from build123d import *

# Parameters (mm, degrees)
F0_W     = 254
F0_H     = 254
F1_DEPTH = 82.87358
F4_R     = 13.060022
F5_DEPTH = 44.433


with BuildPart() as f1:
    # F0 (on Top) → F1 (new body)
    with BuildSketch(Plane.XY):
        Rectangle(F0_W, F0_H)
    extrude(amount=F1_DEPTH)


with BuildPart() as f3:
    # F2 (on Right) → F3 (revolve)
    with BuildSketch(Plane.YZ):
        Polygon((-27.195146, 7.24093), (-35.484381, 0), (42.802874, 0), (42.802874, 21.363337), (-8.774616, 21.363337), (-14.914793, 7.24093), align=None)
    revolve(axis=Axis((0, 3.659246, 0), (0, -1, 0)))


with BuildPart() as f5_tool:
    # F4 (on face) → F5 (new body)
    with BuildSketch(Plane(origin=(0, 42.802874, 0), x_dir=(-1, 0, 0), z_dir=(0, 1, 0))):
        Circle(F4_R)
    extrude(amount=-F5_DEPTH)


with BuildPart() as f1_1:
    add(f1.part)

    # F5: cut by f5_tool
    add(f5_tool.part, mode=Mode.SUBTRACT)


with BuildPart() as f3_1:
    add(f3.part)

    # F5: cut by f5_tool
    add(f5_tool.part, mode=Mode.SUBTRACT)


with BuildPart() as f1_2:
    add(f1_1.part)

    # F6: intersect F3
    add(f3_1.part, mode=Mode.INTERSECT)


solid = f1_2.part
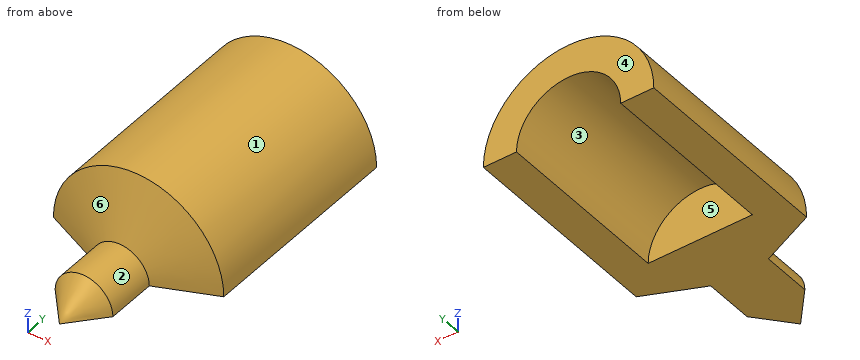
Verification items for the finished model (mm, model axes). Face numbers are marked on the shaded views. A direction names the side the tool comes from. Give positions to 0.01 mm unless a question says otherwise; leave off trailing zeros. Write each loop counter-clockwise with the first axis right and the second up, starting at its lowest first coordinate (ties: lowest second). Pieces come first, ordered by that corner, then holes.
(1) Cross-section at A-A (x = 0). Enter the section's corners in (y, z).
(2) Access from +Z, -Z, +X, -X, +Y, -Y to the whole of each face (thin tool, end or side, straight path). Record for the marked faces 1, 2 and 3.
(3) Gauge pin test, flat ends, axial feed: pin 1 (12 mm diameter, centred on x = 10, y = 2, fed in from +Z); pin 2 (2 mm diameter, centred on y = -12, z = 4, fed in from +X); pin 3 (6 mm diameter, centred on x = 0, z = 14.5, fed in from -Y). Record the tip position at first contact, or that the pin passes through.
(4) Material ranges on line 1 (X direction, y = 27.5, z = 11.5); line 2 (X direction, y = 34, z = 7.5); line 3 (X direction, y = -28.5, z = 5), recorded low to high.
(5) Cross-section at B-B (y = -2.5). Enter the section's corners in (x, z), plus the area to 3 significant figures.
(6) Mould release check, pull along X, two halves, no side actions. Record for the marked faces 4, 5 and 6: +X half, -X half, draft (parallel to the pull), parting line (faces both ways), or undercut.
Worked out:
1. outline: (-35.48, 0) - (-1.63, 0) - (-1.63, 13.06) - (42.8, 13.06) - (42.8, 21.36) - (-8.77, 21.36) - (-14.91, 7.24) - (-27.2, 7.24) - close
2. face 1: +Z, +Y, -Y
2. face 2: +Z, -Y
2. face 3: -Z, +Y
3. pin 1: stops at z = 20.99
3. pin 2: stops at x = 15.76
3. pin 3: stops at y = -13.06
4. line 1: x = -18 to -6.19, 6.19 to 18
4. line 2: x = -20 to -10.69, 10.69 to 20
4. line 3: x = -3.5 to 3.5
5. outline: (-21.36, 0) - (21.36, 0) arc R21.36 ccw to start
5. area: 717 mm2
6. face 4: draft
6. face 5: undercut
6. face 6: parting line
